from build123d import *

# Parameters (mm, degrees)
SKETCH1_R           = 14.29
SKETCH1_R_2         = 2.5
BOSS_EXTRUDE1_DEPTH = 4


with BuildPart() as part:
    # Sketch1 → Boss-Extrude1 (new body)
    with BuildSketch(Plane.XY):
        with BuildLine():
            Line((42.153928026, 12.438673777), (23.259125181, -1.491803793))
            ThreePointArc((23.259125181, -1.491803793), (21.087687699, -3.684227098), (19.688057389, -6.434299039))
            ThreePointArc((19.688057389, -6.434299039), (17.183961156, -11.564224439), (13.374639809, -15.815777498))
            ThreePointArc((13.374639809, -15.815777498), (-5.55728281, -19.953356), (-19.624705783, -6.625007986))
            ThreePointArc((-19.624705783, -6.625007986), (-20.997947453, -3.961204504), (-23.098831149, -1.823933026))
            Line((-23.098831149, -1.823933026), (-42.200396688, 12.504304927))
            ThreePointArc((-42.200396688, 12.504304927), (-44.261108051, 14.973735796), (-45.00000949, 18.104014507))
            Line((-45.00000949, 18.104014507), (-45.00000949, 85.67919791))
            Line((-45.00000949, 85.67919791), (-45.00000949, 92.880351926))
            Line((-45.00000949, 92.880351926), (44.99999051, 92.880351926))
            Line((44.99999051, 92.880351926), (44.99999051, 90.002365232))
            Line((44.99999051, 90.002365232), (44.99999051, 18.072926444))
            ThreePointArc((44.99999051, 18.072926444), (44.248092726, 14.916786603), (42.153928026, 12.438673777))
        make_face()
        Circle(SKETCH1_R, mode=Mode.SUBTRACT)
        with Locations((0, 64.87)):
            Circle(SKETCH1_R, mode=Mode.SUBTRACT)
        with Locations((37.99999051, 48.238911282)):
            Circle(SKETCH1_R_2, mode=Mode.SUBTRACT)
        with Locations((37.99999051, 71.343473564)):
            Circle(SKETCH1_R_2, mode=Mode.SUBTRACT)
        with Locations(Location((-37.99999051, 48.238911282, 0), (0, 0, 180))):
            Circle(SKETCH1_R_2, mode=Mode.SUBTRACT)
        with Locations(Location((-37.99999051, 71.343473564, 0), (0, 0, 180))):
            Circle(SKETCH1_R_2, mode=Mode.SUBTRACT)
        with BuildLine():
            Line((13.574400229, 44.968526689), (30.750314435, 22.722318802))
            ThreePointArc((30.750314435, 22.722318802), (31.147959551, 21.222946572), (30.35409022, 19.890276241))
            Line((30.35409022, 19.890276241), (20.739573812, 12.80182942))
            ThreePointArc((20.739573812, 12.80182942), (19.25353688, 12.434122338), (17.942793433, 13.224986345))
            ThreePointArc((17.942793433, 13.224986345), (-0.05305295, 22.289936864), (-18.005544161, 13.139424624))
            ThreePointArc((-18.005544161, 13.139424624), (-19.325388182, 12.340361548), (-20.821226271, 12.718460012))
            Line((-20.821226271, 12.718460012), (-30.377654795, 19.886813915))
            ThreePointArc((-30.377654795, 19.886813915), (-31.159381655, 21.217806836), (-30.760607673, 22.708987023))
            Line((-30.760607673, 22.708987023), (-13.574400229, 44.968526689))
            ThreePointArc((-13.574400229, 44.968526689), (-12.385736887, 45.706997131), (-11.003989114, 45.485564914))
            ThreePointArc((-11.003989114, 45.485564914), (0, 42.58), (11.003989114, 45.485564914))
            ThreePointArc((11.003989114, 45.485564914), (12.385736887, 45.706997131), (13.574400229, 44.968526689))
        make_face(mode=Mode.SUBTRACT)
        with BuildLine():
            Line((21.895204833, 77.38684864), (24.99999051, 77.38684864))
            ThreePointArc((24.99999051, 77.38684864), (29.949737978, 75.336596108), (31.99999051, 70.38684864))
            Line((31.99999051, 70.38684864), (31.99999051, 48.238911282))
            ThreePointArc((31.99999051, 48.238911282), (30.645696708, 46.346013105), (28.416927004, 47.016655197))
            Line((28.416927004, 47.016655197), (21.474414878, 56.008582273))
            ThreePointArc((21.474414878, 56.008582273), (21.085896999, 56.894881748), (21.158962255, 57.859834788))
            ThreePointArc((21.158962255, 57.859834788), (22.244467277, 66.293999852), (20.092388461, 74.520908036))
            ThreePointArc((20.092388461, 74.520908036), (20.202295915, 76.451770889), (21.895204833, 77.38684864))
        make_face(mode=Mode.SUBTRACT)
        with BuildLine():
            Line((-31.99999051, 70.38684864), (-31.99999051, 48.238911282))
            ThreePointArc((-31.99999051, 48.238911282), (-30.645696708, 46.346013105), (-28.416927004, 47.016655197))
            Line((-28.416927004, 47.016655197), (-21.474414878, 56.008582273))
            ThreePointArc((-21.474414878, 56.008582273), (-21.085896999, 56.894881748), (-21.158962255, 57.859834788))
            ThreePointArc((-21.158962255, 57.859834788), (-22.244467277, 66.293999852), (-20.092388461, 74.520908036))
            ThreePointArc((-20.092388461, 74.520908036), (-20.202295915, 76.451770889), (-21.895204833, 77.38684864))
            Line((-21.895204833, 77.38684864), (-24.99999051, 77.38684864))
            ThreePointArc((-24.99999051, 77.38684864), (-29.949737978, 75.336596108), (-31.99999051, 70.38684864))
        make_face(mode=Mode.SUBTRACT)
    extrude(amount=BOSS_EXTRUDE1_DEPTH)


solid = part.part
Geometry check sheet. Reference: the model listing, model coordinates, mm. A direction names the side the tool comes from. Give positions to 0.01 mm unless a question says otherwise; leave off trailing zeros. Loops run counter-clockwise (first coordinate to the right, second up) from the corner with the lowest first, then second, coordinate; pieces in that order, holes last. Notation, with made-up numbers: M -24,4.25 L -9,4.25 A7 ccw -9,16.25 Z; hole C 28,42.5 d7. An arc over 180 degrees is marked long. Answer as a JSON object with one key per item and string values. Group by question number.
Item 1: Access from +Z, -Z, +X, -X, +Y, -Y to the whole of each face (thin tool, end or side, straight path). Record for faces 4 (the flat face through (-32.516, 5.24, 1.972)), 5 (the cylindrical face through (-12.41, 45.7, 1.97)).
Item 2: Sectioned sample at B-B on x = 0. Record the boundary of the cut face in (y, z), plus the area to 3 significant figures.
Item 3: Gauge pin test, flat ends, axial feed: pin 1 (2 mm diameter, centred on x = 14, y = 40, fed in from -Z); pin 2 (8 mm diameter, centred on x = 27.5, y = 74, fed in from -Z); pin 3 (0.9 mm diameter, centred on x = -24, z = 2, fed in from -Y); pin 4 (1.6 mm diameter, centred on x = 23.5, z = 2.5, fed in from -Y). Record the tip position at first contact, or that the pin passes through.
Item 4: Material ranges on L1, parallel to Y at x = 0, z = 1.75; L2, parallel to Y at x = 30, z = 0.65; L3, parallel to X at y = 52, z = 3.7, recorded low to high.
Item 5: Sectioned sample at C-C on x = -38. Record the boundary of the cut face in (y, z), plus the area to 3 significant figures.
Item 6: Mould release check, pull along Y, two halves, no side actions. Record for faces 1 (the cylindrical face through (44.27, 14.96, 1.97)), 2 (the flat face through (1, 50, 4)), 3 (the flat face through (24.994, 51.45, 1.972)): pulls with the +Y half, pulls with the -Y half, needs draft (parallel to the pull), parting line crosses it, or undercut.
Item 7: Sectioned sample at D-D on y = 10. Record the boundary of the cut face in (x, z).
Item 8: Sectioned sample at A-A on y = 64.87. Record the boundary of the cut face in (x, z), plus the area to 3 significant figures.
Findings below:
{
 "1": {"face 4": "+Z, -Z, -X, -Y", "face 5": "+Z, -Z"},
 "2": {"outline": "M -20.71,0 L -14.29,0 L -14.29,4 L -20.71,4 Z; M 14.29,0 L 22.29,0 L 22.29,4 L 14.29,4 Z; M 42.58,0 L 50.58,0 L 50.58,4 L 42.58,4 Z; M 79.16,0 L 92.88,0 L 92.88,4 L 79.16,4 Z", "area": "145 mm2"},
 "3": {"pin 1": "through", "pin 2": "z = 0", "pin 3": "y = -1.49", "pin 4": "y = -1.94"},
 "4": {"L1": "-20.71 to -14.29, 14.29 to 22.29, 42.58 to 50.58, 79.16 to 92.88", "L2": "3.48 to 19.63, 23.69 to 46.24, 75.29 to 92.88", "L3": "-45 to -32, -24.57 to -6.21, 6.21 to 24.57, 32 to 45"},
 "5": {"outline": "M 9.35,0 L 45.74,0 L 45.74,4 L 9.35,4 Z; M 50.74,0 L 68.84,0 L 68.84,4 L 50.74,4 Z; M 73.84,0 L 92.88,0 L 92.88,4 L 73.84,4 Z", "area": "294 mm2"},
 "6": {"face 1": "pulls with the -Y half", "face 2": "needs draft", "face 3": "undercut"},
 "7": {"outline": "M -38.86,0 L -10.21,0 L -10.21,4 L -38.86,4 Z; M 10.21,0 L 38.85,0 L 38.85,4 L 10.21,4 Z"},
 "8": {"outline": "M -45,0 L -32,0 L -32,4 L -45,4 Z; M -22.29,0 L -14.29,0 L -14.29,4 L -22.29,4 Z; M 14.29,0 L 22.29,0 L 22.29,4 L 14.29,4 Z; M 32,0 L 45,0 L 45,4 L 32,4 Z", "area": "168 mm2"}
}
